```python
from build123d import *

# Parameters (mm, degrees)
EXTRUDE_1_DEPTH     = 12
SKETCH_2_R          = 5
CUT_EXTRUDE_1_DEPTH = 131.40645681
SKETCH_3_R          = 25
EXTRUDE_2_DEPTH     = 25
SKETCH_4_R          = 16
CUT_EXTRUDE_2_DEPTH = 136.021642627
CUT_EXTRUDE_3_DEPTH = 12


with BuildPart() as part:
    # 草圖1 → 填料-伸長1 (new body)
    with BuildSketch(Plane.XY):
        with BuildLine():
            ThreePointArc((25, 95), (0, 120), (-25, 95))
            ThreePointArc((-25, 95), (-29.667879628, 58.377168991), (-43.373037686, 24.096132048))
            ThreePointArc((-43.373037686, 24.096132048), (0, -49.616972679), (43.373037686, 24.096132048))
            ThreePointArc((43.373037686, 24.096132048), (29.667879628, 58.377168991), (25, 95))
        make_face()
        with BuildLine():
            Line((-11, 95), (-11, 53))
            ThreePointArc((-11, 53), (0, 42), (11, 53))
            Line((11, 53), (11, 95))
            ThreePointArc((11, 95), (0, 106), (-11, 95))
        make_face(mode=Mode.SUBTRACT)
    extrude(amount=EXTRUDE_1_DEPTH)

    # 草圖2 → 除料-伸長1 (cut, through all)
    with BuildSketch(Plane.XY.offset(12)):
        with Locations((38, 0)):
            Circle(SKETCH_2_R)
        with Locations((-38, 0)):
            Circle(SKETCH_2_R)
        with Locations((-26.870057685, -26.870057685)):
            Circle(SKETCH_2_R)
        with Locations((0, -38)):
            Circle(SKETCH_2_R)
        with Locations((26.870057685, -26.870057685)):
            Circle(SKETCH_2_R)
    extrude(amount=-CUT_EXTRUDE_1_DEPTH, mode=Mode.SUBTRACT)

    # 草圖3 → 填料-伸長2 (add)
    with BuildSketch(Plane.XY.offset(12)):
        Circle(SKETCH_3_R)
    extrude(amount=EXTRUDE_2_DEPTH)

    # 草圖4 → 除料-伸長2 (cut, through all)
    with BuildSketch(Plane.XY.offset(37)):
        Circle(SKETCH_4_R)
    extrude(amount=-CUT_EXTRUDE_2_DEPTH, mode=Mode.SUBTRACT)

    # 草圖5 → 除料-伸長3 (cut)
    with BuildSketch(Plane.XY.offset(37)):
        with BuildLine():
            Line((-24.494897428, 5), (-15.198684154, 5))
            ThreePointArc((-15.198684154, 5), (-16, 0), (-15.198684154, -5))
            Line((-15.198684154, -5), (-24.494897428, -5))
            ThreePointArc((-24.494897428, -5), (-25, 0), (-24.494897428, 5))
        make_face()
        with BuildLine():
            Line((15.198684154, -5), (24.494897428, -5))
            ThreePointArc((24.494897428, -5), (25, 0), (24.494897428, 5))
            Line((24.494897428, 5), (15.198684154, 5))
            ThreePointArc((15.198684154, 5), (16, 0), (15.198684154, -5))
        make_face()
    extrude(amount=-CUT_EXTRUDE_3_DEPTH, mode=Mode.SUBTRACT)


solid = part.part
```
Here's how the part is built. I have some questions about the finished solid (model axes, mm). A direction names the side the tool comes from. Coordinates: 2 decimals unless noted, no trailing zeros. Order: outer loops, then holes, each group sorted by start corner. A loop starts at its lowest first (then second) coordinate and runs counter-clockwise, first axis right, second up. Notation, with made-up numbers: (43, 1.5) - (60, 1.5) arc R20 cw to (60, 8.5) - close; hole circle Ø7 at (64, -36.5). An arc over 180 degrees is marked (long way). One line per question, with ' | ' between items. Start each with the question number.
1. Which directions (+Z, -Z, +X, -X, +Y, -Y) give clear straight access to the entire face, cutting with the end or side of a thin tool? Please do faces 1 (the flat face through (-20, 5, 31)), 2 (the flat face through (0, -17, 37)), 3 (the cylindrical face through (0, 42, 6)).
2. If we section it at A-A (x = 0): Write out the boundary of the cut face in (y, z), and give its area (3 significant figures).
3. If we mould it in two halves opening along X, with no side actions, what happens to faces 4 (the flat face through (11, 74, 6)), 5 (the cylindrical face through (23.09, -9.58, 24.32)), 6 (the flat face through (-20, -5, 31)), 7 (the cylindrical face through (3, -34, 6))? For each: released by +X, released by -X, zero draft, split by the parting line, or undercut.
4. Please list where these lines run through material, in increasing order: line 1 along Y through (x, z) = (0, 9.25); line 2 along Y through (x, z) = (0, 14.5). Write a range as [from, to].
5. I'm going to push flat-ended pins straight in: pin 1 Ø8 at (x, y) = (38, 0) entering from +Z; pin 2 Ø7.5 at (x, z) = (-19.5, 32) entering from -Y; pin 3 Ø7.5 at (x, z) = (17.5, 32) entering from +Y; pin 4 Ø3 at (x, y) = (-18.5, -1) entering from +Z. Where does each tip first touch, or does it pass through?
6. If we section it at D-D (y = -38): Write out the boundary of the cut face in (x, z), and give its area (3 significant figures).
7. If we section it at B-B (y = 0): Write out the boundary of the cut face in (x, z).
8. If we section it at C-C (z = 8): Write out the boundary of the cut face in (x, y).
Model answer:
1) face 1: +Z, +X, -X | face 2: +Z, +X, -X, +Y, -Y | face 3: +Z, -Z
2) outline: (-49.62, 0) - (-43, 0) - (-43, 12) - (-49.62, 12) - close; (-33, 0) - (-16, 0) - (-16, 37) - (-25, 37) - (-25, 12) - (-33, 12) - close; (16, 0) - (42, 0) - (42, 12) - (25, 12) - (25, 37) - (16, 37) - close; (106, 0) - (120, 0) - (120, 12) - (106, 12) - close | area: 1,210 mm²
3) face 4: undercut | face 5: split by the parting line | face 6: zero draft | face 7: undercut
4) line 1: y = [-49.62, -43], [-33, -16], [16, 42], [106, 120] | line 2: y = [-25, -16], [16, 25]
5) pin 1: passes through | pin 2: stops at y = -19.41 | pin 3: stops at y = 20.88 | pin 4: stops at z = 25
6) outline: (-31.9, 0) - (-5, 0) - (-5, 12) - (-31.9, 12) - close; (5, 0) - (31.9, 0) - (31.9, 12) - (5, 12) - close | area: 646 mm²
7) outline: (-49.62, 0) - (-43, 0) - (-43, 12) - (-49.62, 12) - close; (-33, 0) - (-16, 0) - (-16, 25) - (-25, 25) - (-25, 12) - (-33, 12) - close; (16, 0) - (33, 0) - (33, 12) - (25, 12) - (25, 25) - (16, 25) - close; (43, 0) - (49.62, 0) - (49.62, 12) - (43, 12) - close
8) outline: (-43.37, 24.1) arc R49.62 ccw (long way) to (43.37, 24.1) arc R146 cw to (25, 95) arc R25 ccw to (-25, 95) arc R146 cw to start; hole circle Ø10 at (-38, 0); hole circle Ø10 at (-26.87, -26.87); hole circle Ø32 at (0, 0); hole (-11, 53) arc R11 ccw to (11, 53) - (11, 95) arc R11 ccw to (-11, 95) - close; hole circle Ø10 at (0, -38); hole circle Ø10 at (26.87, -26.87); hole circle Ø10 at (38, 0)
